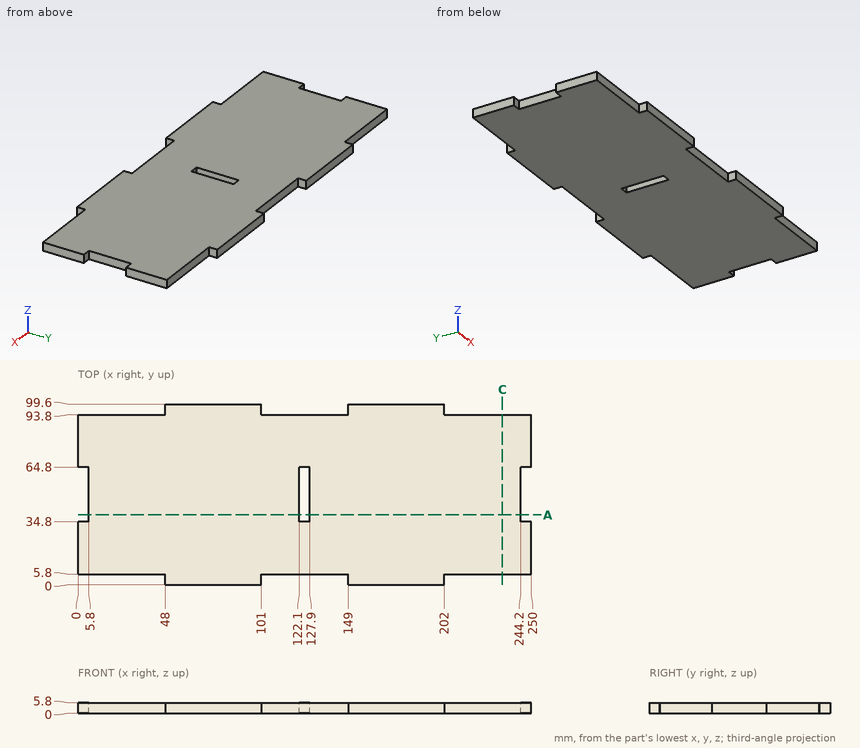
Can you work these out from the drawing? Everything is in mm from the part's minimum corner. Coordinates: 2 decimals unless noted, no trailing zeros. Loops run counter-clockwise (first coordinate to the right, second up) from the corner with the lowest first, then second, coordinate; pieces in that order, holes last.
1. Imagine slicing it at C-C, the plane x = 234. Please give me the cut outline in (y, z).
2. Imagine slicing it at A-A, the plane y = 38.5. Please give me the cut outline in (x, z).
3. I need wall thicknesses on L1, parallel to X at y = 50, z = 1.9; L2, parallel to X at y = 95, z = 2.55; L3, parallel to Y at x = 43, z = 1.2. Which ranges of each line are inside material? Lowest first, please.
4. For P1, Ø1.7, axis at x = 4, z = 3.5, coming from the -Y side; P2, Ø1.7, axis at y = 97.5, z = 3.5, coming from the -X side; P3, Ø1.7, axis at y = 55.5, z = 2.5, coming from the -X side, each with a flat end and sliding along its axis, tell me the tip position at first contact or that it passes through.
Taken from the geometry:
1. outline: (5.8, 0) - (93.8, 0) - (93.8, 5.8) - (5.8, 5.8) - close
2. outline: (5.8, 0) - (122.1, 0) - (122.1, 5.8) - (5.8, 5.8) - close; (127.9, 0) - (244.2, 0) - (244.2, 5.8) - (127.9, 5.8) - close
3. L1: x = 5.8 to 122.1, 127.9 to 244.2
3. L2: x = 48 to 101, 149 to 202
3. L3: y = 5.8 to 93.8
4. P1: stops at y = 5.8
4. P2: stops at x = 48
4. P3: stops at x = 5.8
